Could you check a few things on this drawing? It's one solid part, dimensions in mm from its lowest x, y, z. Round coordinates to 2 decimals unless told otherwise and drop trailing zeros. Write each loop counter-clockwise with the first axis right and the second up, starting at its lowest first coordinate (ties: lowest second). Pieces come first, ordered by that corner, then holes. Notation, with made-up numbers: (78, 7) - (110, 7) arc R21 ccw to (110, 25) - close; hole circle Ø8 at (82.5, 58). An arc over 180 degrees is marked (long way). Use one line per item in the form item = value. Start each with the question number.
1. I want a section at D-D, the plane y = 21. List the corners of the cut face in (x, z) for me.
2. I want a section at B-B, the plane z = 1.1. List the corners of the cut face in (x, y) for me, plus the area to 3 significant figures.
3. If I drill on line 1 along X through (y, z) = (5, 0.95); line 2 along Y through (x, z) = (67, 1.45); line 3 along Y through (x, z) = (61.5, 1.25), over which ranges is the centre line in solid material (lowest first)?
4. I want a section at A-A, the plane y = 5. List the corners of the cut face in (x, z) for me, plus the area to 3 significant figures.
5. I want a section at C-C, the plane x = 5. List the corners of the cut face in (y, z) for me.
6. Will these pins go through, and if not, where does the flat tip stop? pin 1 (4 mm diameter, centred on x = 33, y = 20, fed in from -Z); pin 2 (1 mm diameter, centred on x = 7.5, z = 1.5, fed in from +Y).
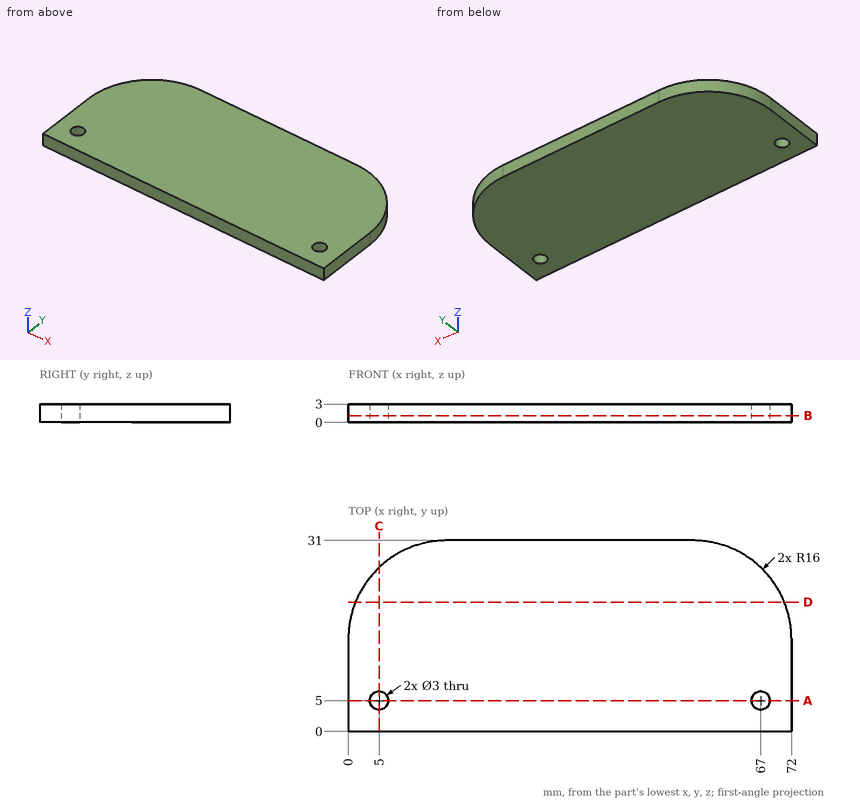
Model answer:
q1.outline = (1.17, 0) - (70.83, 0) - (70.83, 3) - (1.17, 3) - close
q2.outline = (0, 0) - (72, 0) - (72, 15) arc R16 ccw to (56, 31) - (16, 31) arc R16 ccw to (0, 15) - close; hole circle Ø3 at (5, 5); hole circle Ø3 at (67, 5)
q2.area = 2,110 mm2
q3.line_1 = 0 to 3.5, 6.5 to 65.5, 68.5 to 72
q3.line_2 = 0 to 3.5, 6.5 to 26.62
q3.line_3 = 0 to 30.02
q4.outline = (0, 0) - (3.5, 0) - (3.5, 3) - (0, 3) - close; (6.5, 0) - (65.5, 0) - (65.5, 3) - (6.5, 3) - close; (68.5, 0) - (72, 0) - (72, 3) - (68.5, 3) - close
q4.area = 198 mm2
q5.outline = (0, 0) - (3.5, 0) - (3.5, 3) - (0, 3) - close; (6.5, 0) - (26.62, 0) - (26.62, 3) - (6.5, 3) - close
q6.pin_1 = 0
q6.pin_2 = 28.86
